For this review, take the finished solid that the model builds, in its own axes (mm). A direction names the side the tool comes from. Round coordinates to 2 decimals unless told otherwise and drop trailing zeros. Loops run counter-clockwise (first coordinate to the right, second up) from the corner with the lowest first, then second, coordinate; pieces in that order, holes last.
1. To check wall thickness, follow line 1 along Z through (x, y) = (-5.25, 1.75); line 2 along X through (y, z) = (1, 3.25); line 3 along Z through (x, y) = (10, 1.75). State the ranges of each line that lie inside material, in increasing order.
2. Draft analysis for pull direction Z (two halves, no side actions). For faces 1 (the cylindrical face through (13.41, 1.26, -9.52)), 2 (the flat face through (11, 2, -5.143)), 3 (the flat face through (-14.7, 1, 0)), state which applies: released by +Z, released by -Z, zero draft, split by the parting line, or undercut.
3. Tool access review of faces 4 (the cylindrical face through (-8.964, 1.04, -6.507)), 5 (the flat face through (11, 2, 7.556)): name each direction out of +Z, -Z, +X, -X, +Y, -Y from which nothing blocks a thin tool from reaching the whole face with its end or side.
4. Consider section C-C on x = -7.75. State the section outline as (y, z) points, then the cut area to 3 significant figures.
5. Consider section A-A on z = -0.75. State the section outline as (x, y) points.
6. Consider section B-B on y = 0.5. State the section outline as (x, z) points.
7. Clearance check with flat-ended pins moving along their axes: pin 1 Ø0.7 at (x, z) = (10.5, -6.5) entering from -Y; pin 2 Ø0.8 at (x, y) = (-11, 2) entering from +Z; pin 3 Ø0.7 at (x, z) = (-12, -6.5) entering from -Y. State where each tip first meets the part, or that it passes through.
from build123d import *

# Parameters (mm, degrees)
BOSS_EXTRUDE1_DEPTH   = 2.55
SKETCH2_R             = 1.2065
BOSS_EXTRUDE2_DEPTH   = 2.5
BOSS_EXTRUDE2_2_DEPTH = 2.5
BOSS_EXTRUDE2_3_DEPTH = 2.5
BOSS_EXTRUDE2_4_DEPTH = 2.5
SKETCH3_W             = 2.550724021
SKETCH3_H             = 2.413
BOSS_EXTRUDE3_DEPTH   = 1


with BuildPart() as part:
    # Sketch1 → Boss-Extrude1 (new body)
    with BuildSketch(Plane(origin=(0, 0, 0), x_dir=(1, 0, 0), z_dir=(0, 1, 0))):
        with BuildLine():
            Line((-14.7, 6.35), (-14.7, -6.35))
            ThreePointArc((-14.7, -6.35), (-13.370264787, -9.560264787), (-10.16, -10.89))
            Line((-10.16, -10.89), (10.16, -10.89))
            ThreePointArc((10.16, -10.89), (13.370264787, -9.560264787), (14.7, -6.35))
            Line((14.7, -6.35), (14.7, 6.35))
            ThreePointArc((14.7, 6.35), (13.370264787, 9.560264787), (10.16, 10.89))
            Line((10.16, 10.89), (-10.16, 10.89))
            ThreePointArc((-10.16, 10.89), (-13.370264787, 9.560264787), (-14.7, 6.35))
        make_face()
        with BuildLine():
            Line((-10.16, 8.89), (10.16, 8.89))
            ThreePointArc((10.16, 8.89), (11.956051224, 8.146051224), (12.7, 6.35))
            Line((12.7, 6.35), (12.7, -6.35))
            ThreePointArc((12.7, -6.35), (11.956051224, -8.146051224), (10.16, -8.89))
            Line((10.16, -8.89), (-10.16, -8.89))
            ThreePointArc((-10.16, -8.89), (-11.956051224, -8.146051224), (-12.7, -6.35))
            Line((-12.7, -6.35), (-12.7, 6.35))
            ThreePointArc((-12.7, 6.35), (-11.956051224, 8.146051224), (-10.16, 8.89))
        make_face(mode=Mode.SUBTRACT)
    extrude(amount=BOSS_EXTRUDE1_DEPTH)



with BuildPart() as body_2:
    # Sketch2 → Boss-Extrude2 (new body)
    with BuildSketch(Plane(origin=(0, 2.55, 0), x_dir=(1, 0, 0), z_dir=(0, 1, 0))):
        with Locations(Location((10.16, 6.35, 0), (0, 0, 270))):
            Circle(SKETCH2_R)
    extrude(amount=-BOSS_EXTRUDE2_DEPTH)


with BuildPart() as body_3:
    # Sketch2 → Boss-Extrude2 2 (new body)
    with BuildSketch(Plane(origin=(0, 2.55, 0), x_dir=(1, 0, 0), z_dir=(0, 1, 0))):
        with Locations(Location((-10.16, 6.35, 0), (0, 0, 270))):
            Circle(SKETCH2_R)
    extrude(amount=-BOSS_EXTRUDE2_2_DEPTH)


with BuildPart() as body_4:
    # Sketch2 → Boss-Extrude2 3 (new body)
    with BuildSketch(Plane(origin=(0, 2.55, 0), x_dir=(1, 0, 0), z_dir=(0, 1, 0))):
        with Locations(Location((-10.16, -6.35, 0), (0, 0, 270))):
            Circle(SKETCH2_R)
    extrude(amount=-BOSS_EXTRUDE2_3_DEPTH)


with BuildPart() as body_5:
    # Sketch2 → Boss-Extrude2 4 (new body)
    with BuildSketch(Plane(origin=(0, 2.55, 0), x_dir=(1, 0, 0), z_dir=(0, 1, 0))):
        with Locations(Location((10.16, -6.35, 0), (0, 0, 270))):
            Circle(SKETCH2_R)
    extrude(amount=-BOSS_EXTRUDE2_4_DEPTH)


with BuildPart() as part_1:
    add(part.part)

    add(body_2.part)  # Boss-Extrude3 merges body 2

    add(body_3.part)  # Boss-Extrude3 merges body 3

    add(body_4.part)  # Boss-Extrude3 merges body 4

    add(body_5.part)  # Boss-Extrude3 merges body 5
    # Sketch3 → Boss-Extrude3 (add)
    with BuildSketch(Plane(origin=(0, 2.55, 0), x_dir=(1, 0, 0), z_dir=(0, 1, 0))):
        with Locations((-11.42463799, 6.349952339)):
            Rectangle(SKETCH3_W, SKETCH3_H)
        with Locations((11.42463799, 6.349952339)):
            Rectangle(SKETCH3_W, SKETCH3_H)
        with Locations((11.42463799, -6.349952339)):
            Rectangle(SKETCH3_W, SKETCH3_H)
        with Locations((-11.42463799, -6.349952339)):
            Rectangle(SKETCH3_W, SKETCH3_H)
    extrude(amount=-BOSS_EXTRUDE3_DEPTH)


solid = part_1.part
Resolved:
1. line 1: z = -10.89 to -8.89, 8.89 to 10.89
1. line 2: x = -14.7 to -12.7, 12.7 to 14.7
1. line 3: z = -10.89 to -8.89, -7.55 to -5.15, 5.15 to 7.55, 8.89 to 10.89
2. face 1: released by -Z
2. face 2: undercut
2. face 3: zero draft
3. face 4: -Y
3. face 5: +Y, -Y
4. outline: (0, -10.89) - (2.55, -10.89) - (2.55, -8.89) - (0, -8.89) - close; (0, 8.89) - (2.55, 8.89) - (2.55, 10.89) - (0, 10.89) - close
4. area: 10.2 mm2
5. outline: (-14.7, 0) - (-12.7, 0) - (-12.7, 2.55) - (-14.7, 2.55) - close; (12.7, 0) - (14.7, 0) - (14.7, 2.55) - (12.7, 2.55) - close
6. outline: (-14.7, -6.35) arc R4.54 ccw to (-10.16, -10.89) - (10.16, -10.89) arc R4.54 ccw to (14.7, -6.35) - (14.7, 6.35) arc R4.54 ccw to (10.16, 10.89) - (-10.16, 10.89) arc R4.54 ccw to (-14.7, 6.35) - close; circle Ø2.41 at (-10.16, -6.35); circle Ø2.41 at (-10.16, 6.35); circle Ø2.41 at (10.16, -6.35); circle Ø2.41 at (10.16, 6.35); hole (-12.7, -6.35) arc R2.54 ccw to (-10.16, -8.89) - (10.16, -8.89) arc R2.54 ccw to (12.7, -6.35) - (12.7, 6.35) arc R2.54 ccw to (10.16, 8.89) - (-10.16, 8.89) arc R2.54 ccw to (-12.7, 6.35) - close
7. pin 1: stops at y = 0.05
7. pin 2: stops at z = 10.87
7. pin 3: stops at y = 1.55
